Geometry check sheet. Reference: the model listing, model coordinates, mm. A direction names the side the tool comes from. Give positions to 0.01 mm unless a question says otherwise; leave off trailing zeros. Write each loop counter-clockwise with the first axis right and the second up, starting at its lowest first coordinate (ties: lowest second). Pieces come first, ordered by that corner, then holes. Notation, with made-up numbers: (-7.5, 60.25) - (2.5, 60.25) arc R18 ccw to (2.5, 82.25) - close; hole circle Ø3 at (43.25, 64). An arc over 180 degrees is marked (long way). Use a Markdown table: item, result.
```python
from build123d import *

# Parameters (mm, degrees)
SKETCH2_R           = 75
SKETCH2_R_2         = 59
SKETCH2_R_3         = 47
BOSS_EXTRUDE1_DEPTH = 8
SKETCH4_R           = 2.5
CUT_EXTRUDE1_DEPTH  = 8
SKETCH5_R           = 1.9
CUT_EXTRUDE2_DEPTH  = 8
SKETCH7_R           = 22.5
CUT_EXTRUDE3_DEPTH  = 3
SKETCH8_R           = 24
SKETCH8_R_2         = 21
BOSS_EXTRUDE3_DEPTH = 32
SKETCH9_R           = 2.5
CUT_EXTRUDE4_DEPTH  = 8
SKETCH10_R          = 2
CUT_EXTRUDE7_DEPTH  = 2


with BuildPart() as part:
    # Sketch1 → Revolve1 (revolve)
    with BuildSketch(Plane(origin=(0, 0, 0), x_dir=(-1, 0, 0), z_dir=(0, 0, -1)), mode=Mode.PRIVATE) as revolve1_sk:
        with BuildLine():
            Line((-59, -1.1276), (-47, -1.1276))
            ThreePointArc((-47, -1.1276), (-46.292893219, -0.834706781), (-46, -0.1276))
            Line((-46, -0.1276), (-46, 5.8724))
            Line((-46, 5.8724), (-47, 6.8724))
            Line((-47, 6.8724), (-49.4043, 6.8724))
            ThreePointArc((-49.4043, 6.8724), (-52.5, 5.8405), (-55.5957, 6.8724))
            Line((-55.5957, 6.8724), (-59, 6.8724))
            Line((-59, 6.8724), (-60, 5.8724))
            Line((-60, 5.8724), (-60, -0.1276))
            ThreePointArc((-60, -0.1276), (-59.707106781, -0.834706781), (-59, -1.1276))
        make_face()
    revolve(revolve1_sk.sketch.rotate(Axis((0, 0, 0), (0, 1, 0)), 270), axis=Axis((0, 0, 0), (0, 1, 0)))

    # Sketch2 → Boss-Extrude1 (add)
    # profile 1 of 2: a face of its own
    with BuildSketch(Plane.XZ.offset(1.1276)):
        with Locations(Location((0, 0, 0), (0, 0, 270))):
            Circle(SKETCH2_R)
        Circle(SKETCH2_R_2, mode=Mode.SUBTRACT)
    # profile 2 of 2: a face of its own
    with BuildSketch(Plane.XZ.offset(1.1276)):
        Circle(SKETCH2_R_3)
    extrude(amount=-BOSS_EXTRUDE1_DEPTH)

    # Sketch4 → Cut-Extrude1 (cut)
    with BuildSketch(Plane.XZ.offset(1.1276)):
        with Locations(Location((0, 0, 0), (0, 0, 270))):
            Circle(SKETCH4_R)
    extrude(amount=-CUT_EXTRUDE1_DEPTH, mode=Mode.SUBTRACT)

    # Sketch5 → Cut-Extrude2 (cut)
    with BuildSketch(Plane.XZ.offset(1.1276)):
        with Locations(Location((0, 17.5, 0), (0, 0, 270))):
            Circle(SKETCH5_R)
        with Locations(Location((17.5, 0, 0), (0, 0, 270))):
            Circle(SKETCH5_R)
        with Locations(Location((0, -17.5, 0), (0, 0, 270))):
            Circle(SKETCH5_R)
        with Locations(Location((-17.5, 0, 0), (0, 0, 270))):
            Circle(SKETCH5_R)
    extrude(amount=-CUT_EXTRUDE2_DEPTH, mode=Mode.SUBTRACT)

    # Sketch7 → Cut-Extrude3 (cut)
    with BuildSketch(Plane.XZ.offset(1.1276)):
        with Locations(Location((0, 0, 0), (0, 0, 270))):
            Circle(SKETCH7_R)
    extrude(amount=-CUT_EXTRUDE3_DEPTH, mode=Mode.SUBTRACT)

    # Sketch8 → Boss-Extrude3 (add)
    with BuildSketch(Plane(origin=(0, 6.8724, 0), x_dir=(1, 0, 0), z_dir=(0, 1, 0))):
        with Locations(Location((0, 0, 0), (0, 0, 270))):
            Circle(SKETCH8_R)
        with Locations(Location((0, 0, 0), (0, 0, 270))):
            Circle(SKETCH8_R_2, mode=Mode.SUBTRACT)
    extrude(amount=BOSS_EXTRUDE3_DEPTH)

    # Sketch9 → Cut-Extrude4 (cut)
    with BuildSketch(Plane.XZ.offset(1.1276)):
        with Locations(Location((0, -67.5, 0), (0, 0, 270))):
            Circle(SKETCH9_R)
        with Locations(Location((-58.456714755, -33.75, 0), (0, 0, 270))):
            Circle(SKETCH9_R)
        with Locations(Location((-58.456714755, 33.75, 0), (0, 0, 270))):
            Circle(SKETCH9_R)
        with Locations(Location((0, 67.5, 0), (0, 0, 270))):
            Circle(SKETCH9_R)
        with Locations(Location((58.456714755, 33.75, 0), (0, 0, 270))):
            Circle(SKETCH9_R)
        with Locations(Location((58.456714755, -33.75, 0), (0, 0, 270))):
            Circle(SKETCH9_R)
    extrude(amount=-CUT_EXTRUDE4_DEPTH, mode=Mode.SUBTRACT)

    # Sketch10 → Cut-Extrude7 (cut)
    with BuildSketch(Plane.XZ.offset(1.1276)):
        with Locations(Location((-15.100458433, 42.880887256, 0), (0, 0, 270))):
            Circle(SKETCH10_R)
        with Locations(Location((21.160611362, 39.745183733, 0), (0, 0, 270))):
            Circle(SKETCH10_R)
        with Locations(Location((-40.950984141, 20.176327665, 0), (0, 0, 270))):
            Circle(SKETCH10_R)
        with Locations(Location((-42.219460081, -16.197959793, 0), (0, 0, 270))):
            Circle(SKETCH10_R)
    extrude(amount=-CUT_EXTRUDE7_DEPTH, mode=Mode.SUBTRACT)


solid = part.part
```
1) Material ranges on L1, parallel to X at y = 4, z = 0; L2, parallel to X at y = 4.5, z = -33.75; L3, parallel to Z at x = -59.5, y = 2, recorded low to high. Write a range as from..to.
Working result:
| item | result |
|---|---|
| L1 | x = -75..-19.4, -15.6..-2.5, 2.5..15.6, 19.4..75 |
| L2 | x = -66.98..-60.96, -55.96..55.96, 60.96..66.98 |
| L3 | z = -45.66..-36.02, -31.48..31.48, 36.02..45.66 |
2) Depth check by flat-ended pin: P1, Ø4.5, axis at x = 0, z = 0, coming from the -Y side; P2, Ø5, axis at x = -40.95, z = 20.18, coming from the -Y side; P3, Ø3.5, axis at x = -15.1, z = 42.88, coming from the +Y side; P4, Ø3, axis at x = -42, z = -16.5, coming from the -Y side. Enter the tip coordinate at first touch or a pass-through.
Working result:
| item | result |
|---|---|
| P1 | passes through |
| P2 | stops at y = -1.13 |
| P3 | stops at y = 6.87 |
| P4 | stops at y = 0.87 |
3) Section check D-D on z = 67.5. Record the boundary of the cut face in (x, y), then the cut area to 3 significant figures.
Working result:
| item | result |
|---|---|
| outline | (-32.69, -1.13) - (-2.5, -1.13) - (-2.5, 6.87) - (-32.69, 6.87) - close; (2.5, -1.13) - (32.69, -1.13) - (32.69, 6.87) - (2.5, 6.87) - close |
| area | 483 mm² |
4) Section check A-A on z = 0. Count the separate pieces of the cut face and the enclosed holes in it, then the cut area to 3 significant figures.
Working result:
| item | result |
|---|---|
| separate pieces | 4 |
| enclosed holes | 0 |
| area | 1,190 mm² |
5) Set-up check for faces 4 (the flat face through (-16, -1.128, 18)), 5 (the cylindrical face through (6.31, 22.65, 20.03)), 6 (the cylindrical face through (-40.53, -0.14, -17.27)): record each of +Z, -Z, +X, -X, +Y, -Y from which the full face is reachable in a straight line by a thin tool's end or side.
Working result:
| item | result |
|---|---|
| face 4 | +Z, -Z, +X, -X, -Y |
| face 5 | +Y |
| face 6 | -Y |
6) Mould release check, pull along X, two halves, no side actions. Record for faces 1 (the flat face through (-21.2, 38.872, -0.1)), 2 (the cylindrical face through (21.761, -0.142, 37.838)), 3 (the cylindrical face through (7.21, 22.65, 22.89)): pulls with the +X half, pulls with the -X half, needs draft (parallel to the pull), parting line crosses it, or undercut.
Working result:
| item | result |
|---|---|
| face 1 | needs draft |
| face 2 | undercut |
| face 3 | parting line crosses it |
7) Section check B-B on y = 9. Record the boundary of the cut face in (x, z).
Working result:
| item | result |
|---|---|
| outline | circle Ø48 at (0, 0); hole circle Ø42 at (0, 0) |
